```python
from build123d import *

# Parameters (mm, degrees)
SKETCH1_R           = 6.5
SKETCH1_R_2         = 4
BOSS_EXTRUDE1_DEPTH = 10
SKETCH2_W           = 3.218226301
SKETCH2_H           = 3
CUT_EXTRUDE1_DEPTH  = 33
SKETCH3_W           = 12
SKETCH3_H           = 4
BOSS_EXTRUDE2_DEPTH = 10
SKETCH4_R           = 1.5
CUT_EXTRUDE2_DEPTH  = 40
CUT_EXTRUDE3_DEPTH  = 3


with BuildPart() as part:
    # Sketch1 → Boss-Extrude1 (new body)
    with BuildSketch(Plane.XY):
        with Locations((-12.315422017, 2.550703256)):
            Circle(SKETCH1_R)
        with Locations((-12.315422017, 2.550703256)):
            Circle(SKETCH1_R_2, mode=Mode.SUBTRACT)
    extrude(amount=BOSS_EXTRUDE1_DEPTH)

    # Sketch2 → Cut-Extrude1 (cut)
    with BuildSketch(Plane.XY.offset(10)):
        with Locations((-17.357309889, 2.432650589)):
            Rectangle(SKETCH2_W, SKETCH2_H)
    extrude(amount=-CUT_EXTRUDE1_DEPTH, mode=Mode.SUBTRACT)

    # Sketch3 → Boss-Extrude2 (add)
    with BuildSketch(Plane.XY.offset(10)):
        with Locations((-21.973550714, -1.067349411)):
            Rectangle(SKETCH3_W, SKETCH3_H)
        with Locations((-22.069116407, 5.932650589)):
            Rectangle(SKETCH3_W, SKETCH3_H)
    extrude(amount=-BOSS_EXTRUDE2_DEPTH)

    # Sketch4 → Cut-Extrude2 (cut)
    with BuildSketch(Plane(origin=(0, 7.932650589, 0), x_dir=(1, 0, 0), z_dir=(0, 1, 0))):
        with Locations(Location((-22.069116407, -5, 0), (0, 0, 180))):
            Circle(SKETCH4_R)
    extrude(amount=-CUT_EXTRUDE2_DEPTH, mode=Mode.SUBTRACT)

    # Sketch5 → Cut-Extrude3 (cut)
    with BuildSketch(Plane(origin=(0, -3.067349411, 0), x_dir=(-1, 0, 0), z_dir=(0, -1, 0))):
        Polygon((19.051149057, -6.669474185), (22.051149057, -8.401524993), (25.051149057, -6.669474185), (25.051149057, -3.20537257), (22.051149057, -1.473321762), (19.051149057, -3.20537257), align=None)
    extrude(amount=-CUT_EXTRUDE3_DEPTH, mode=Mode.SUBTRACT)


solid = part.part
```
Part model, mm, in its own coordinate system. A direction names the side the tool comes from. Round coordinates to 2 decimals unless told otherwise and drop trailing zeros. Loops run counter-clockwise (first coordinate to the right, second up) from the corner with the lowest first, then second, coordinate; pieces in that order, holes last. Notation, with made-up numbers: (-14, 16.5) -> (35, 16.5) arc R8 ccw to (35, 31.5) -> close; hole circle Ø1 at (37.5, -16.75). An arc over 180 degrees is marked (long way). Use one line per item in the form item = value. Start each with the question number.
Item 1: Tool access for faces 5 (the flat face through (-19.051, -2, 5)), 6 (the flat face through (-20.7, 0.933, 6.2)), 7 (the flat face through (-27.974, -1, 5)): list every direction of +Z, -Z, +X, -X, +Y, -Y with a clear straight run to the whole face (end or side of a thin tool).
Item 2: Band-saw the part on D-D (x = -21.25). List the corners of the cut face in (y, z), plus the area to 3 significant figures.
Item 3: Band-saw the part on A-A (z = 5). List the corners of the cut face in (x, y).
Item 4: Drill centre lines: line 1 along Y through (x, z) = (-26.75, 6); line 2 along X through (y, z) = (-0.5, 3.75); line 3 along Y through (x, z) = (-21.75, 7). Where is each one in solid material? Low to high.
Item 5: Band-saw the part on C-C (x = -17.5). List the corners of the cut face in (y, z), plus the area to 3 significant figures.
Item 6: Two-plate mould, pull along Z, no slides. Class faces 1 (the flat face through (-17.1, 4.1, 0)), 2 (the flat face through (-17.1, 4.1, 10)), 3 (the flat face through (-23.57, -1.59, 2.35)), 4 (the flat face through (-28.069, 6, 5)): released by +Z, released by -Z, zero draft, split by the parting line, or undercut.
Item 7: Band-saw the part on B-B (y = 5.25). List the corners of the cut face in (x, z), plus the area to 3 significant figures.
Item 8: Drop flat-ended pins along their axis: pin 1 Ø3.5 at (y, z) = (-1.5, 6) entering from -X; pin 2 Ø3 at (x, y) = (-25.5, 5) entering from -Z; pin 3 Ø3.5 at (x, z) = (-22.07, 5) entering from +Y; pin 4 Ø1 at (y, z) = (-0.5, 3.5) entering from +X. Give the stop position or say it passes through.
Data:
q1.face_5 = -Y
q1.face_6 = +Z, -Z, -X
q1.face_7 = +Z, -Z, -X, -Y
q2.outline = (-3.07, 0) -> (0.93, 0) -> (0.93, 3.74) -> (-0.07, 3.74) -> (-0.07, 1.94) -> (-3.07, 1.94) -> close; (-3.07, 7.94) -> (-0.07, 7.94) -> (-0.07, 6.26) -> (0.93, 6.26) -> (0.93, 10) -> (-3.07, 10) -> close; (3.93, 0) -> (7.93, 0) -> (7.93, 3.74) -> (3.93, 3.74) -> close; (3.93, 6.26) -> (7.93, 6.26) -> (7.93, 10) -> (3.93, 10) -> close
q2.area = 49.4 mm^2
q3.outline = (-28.07, 3.93) -> (-23.57, 3.93) -> (-23.57, 7.93) -> (-28.07, 7.93) -> close; (-27.97, -3.07) -> (-25.05, -3.07) -> (-25.05, -0.07) -> (-23.57, -0.07) -> (-23.57, 0.93) -> (-27.97, 0.93) -> close; (-20.57, -0.07) -> (-19.05, -0.07) -> (-19.05, -3.07) -> (-15.97, -3.07) -> (-15.97, -2.82) arc R6.5 ccw (long way) to (-16.07, 7.86) -> (-16.07, 7.93) -> (-20.57, 7.93) -> (-20.57, 3.93) -> (-16.07, 3.93) arc R4 cw (long way) to (-15.97, 0.93) -> (-20.57, 0.93) -> close
q4.line_1 = -3.07 to 0.93, 3.93 to 7.93
q4.line_2 = -27.97 to -25.05, -19.05 to -14.9, -9.73 to -6.58
q4.line_3 = -0.07 to 0.93, 3.93 to 7.93
q5.outline = (-3.07, 0) -> (0.93, 0) -> (0.93, 10) -> (-3.07, 10) -> close; (3.93, 0) -> (7.93, 0) -> (7.93, 10) -> (3.93, 10) -> close
q5.area = 80.0 mm^2
q6.face_1 = released by -Z
q6.face_2 = released by +Z
q6.face_3 = undercut
q6.face_4 = zero draft
q7.outline = (-28.07, 0) -> (-15.27, 0) -> (-15.27, 10) -> (-28.07, 10) -> close; (-9.36, 0) -> (-6.4, 0) -> (-6.4, 10) -> (-9.36, 10) -> close; hole circle Ø3 at (-22.07, 5)
q7.area = 151 mm^2
q8.pin_1 = -27.97
q8.pin_2 = 0
q8.pin_3 = 7.93
q8.pin_4 = -6.34
